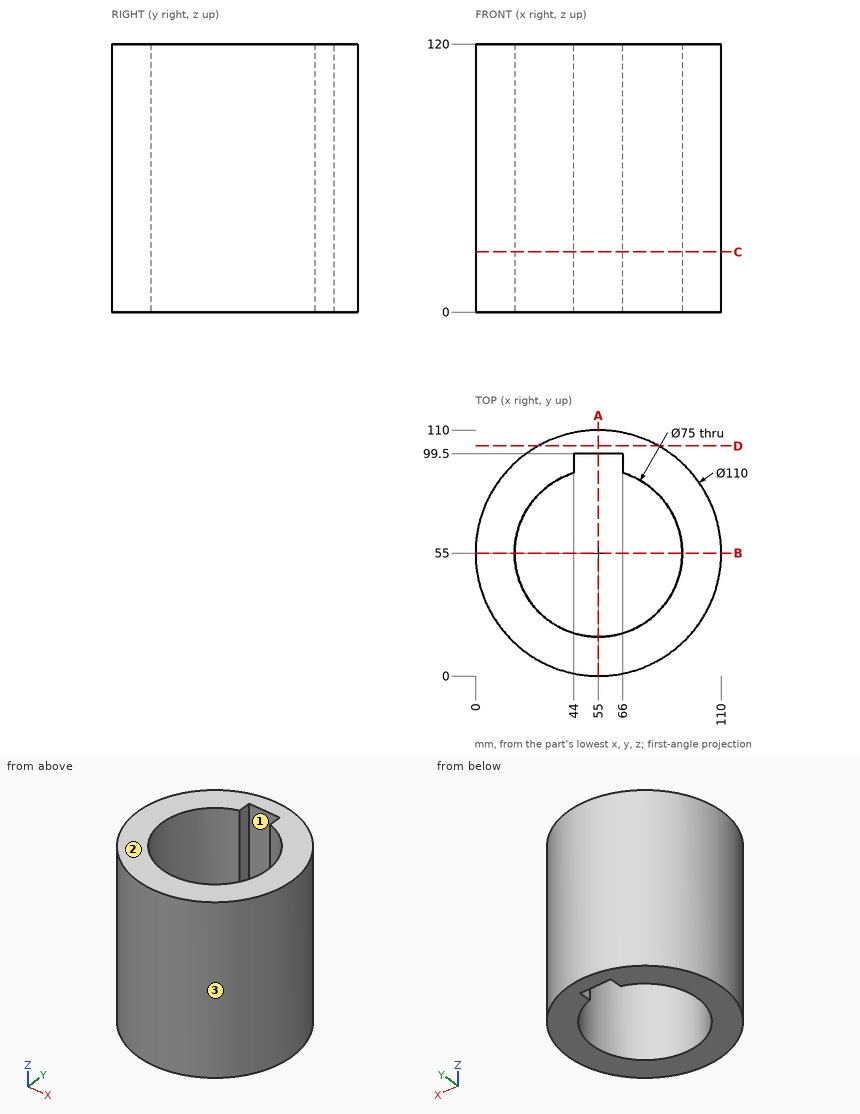
Input: dimensioned drawing with shaded views. Units: mm. Origin: part minimum x, y, z. Give positions to 0.01 mm unless a question says otherwise; leave off trailing zeros. Write each loop counter-clockwise with the first axis right and the second up, starting at its lowest first coordinate (ties: lowest second). Pieces come first, ordered by that corner, then holes. Notation, with made-up numbers: (69.5, -30) - (87.5, -30) arc R8 ccw to (87.5, -17) - close; hole circle Ø5 at (-27.75, -19). An arc over 180 degrees is marked (long way). Write item = value, one per line. Start each with the question number.
1) Draft query along Y for the marked faces 1, 2 and 3. Return one class per face: pulls with the +Y half, pulls with the -Y half, needs draft (parallel to the pull), parting line crosses it, or undercut.
2) Cut plane D-D (y = 103). Return loops of the section in (x, z).
3) Cut plane B-B (y = 55). Return loops of the section in (x, z).
4) Cut plane A-A (x = 55). Return loops of the section in (y, z).
5) Pin query (flat end, axial travel): pin 1 (4 mm diameter, centred on x = 31.5, z = 66.5, fed in from -Y); pin 2 (12 mm diameter, centred on y = 13.5, z = 25, fed in from +X); pin 3 (11 mm diameter, centred on x = 58, z = 84, fed in from -Y). Return the tip coordinate at first contact, or that it passes through.
6) Cut plane C-C (z = 27). Return loops of the section in (x, y).
7) Material intervals for L1, parallel to Y at x = 55, z = 87; L2, parallel to Y at x = 46, z = 36.5; L3, parallel to X at y = 96, z = 51, sorted ascending. Write a range as [from, to].
Answers follow:
q1.face_1 = undercut
q1.face_2 = needs draft
q1.face_3 = parting line crosses it
q2.outline = (28.15, 0) - (81.85, 0) - (81.85, 120) - (28.15, 120) - close
q3.outline = (0, 0) - (17.5, 0) - (17.5, 120) - (0, 120) - close; (92.5, 0) - (110, 0) - (110, 120) - (92.5, 120) - close
q4.outline = (0, 0) - (17.5, 0) - (17.5, 120) - (0, 120) - close; (99.5, 0) - (110, 0) - (110, 120) - (99.5, 120) - close
q5.pin_1 = 4.38
q5.pin_2 = 97.01
q5.pin_3 = 0
q6.outline = circle Ø110 at (55, 55); hole (44, 90.85) arc R37.5 ccw (long way) to (66, 90.85) - (66, 99.5) - (44, 99.5) - close
q7.L1 = [0, 17.5], [99.5, 110]
q7.L2 = [0.74, 18.6], [99.5, 109.26]
q7.L3 = [18.34, 44], [66, 91.66]
